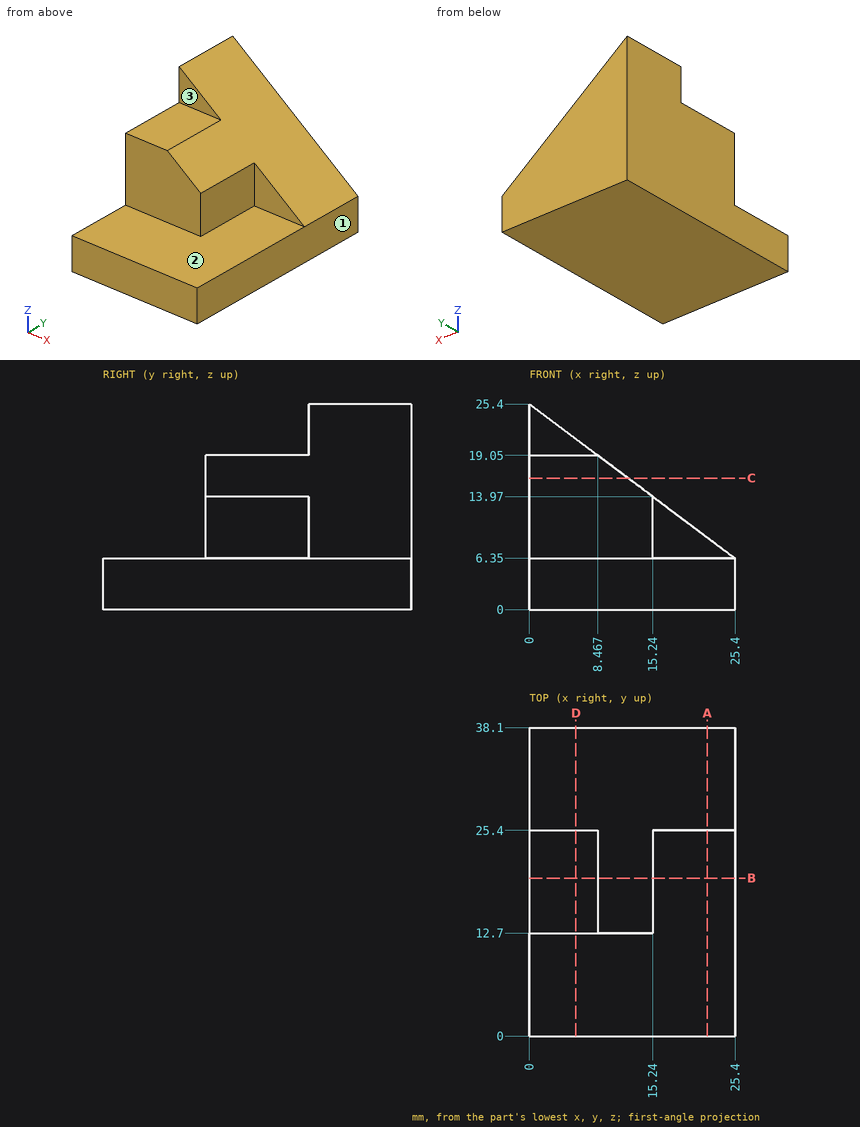
Could you check a few things on this drawing? It's one solid part, dimensions in mm from its lowest x, y, z. A direction names the side the tool comes from. Coordinates: 2 decimals unless noted, no trailing zeros. Loops run counter-clockwise (first coordinate to the right, second up) from the corner with the lowest first, then second, coordinate; pieces in that order, holes last. Notation, with made-up numbers: (89, 76.5) - (110, 76.5) arc R6 ccw to (110, 82.5) - close; hole circle Ø3 at (20, 43). An arc over 180 degrees is marked (long way). Return JSON: item names as keys, results as strings. Group by question number.
Item 1: If we section it at D-D on x = 5.75: Write out the boundary of the cut face in (y, z).
Item 2: Will these pins go through, and if not, where does the flat tip stop? P1, Ø7, axis at x = 4.5, z = 21.5, coming from the -Y side; P2, Ø3, axis at x = 13, y = 10, coming from the +Z side; P3, Ø7, axis at x = 5, y = 19.5, coming from the +Z side.
Item 3: If we section it at C-C on z = 16.25: Write out the boundary of the cut face in (x, y), and give its area (3 significant figures).
Item 4: I need wall thicknesses on line 1 (Y direction, x = 2.5, z = 8.5); line 2 (Z direction, x = 5.25, y = 7); line 3 (Z direction, x = 7.75, y = 16.5). Which ranges of each line are inside material? Lowest first, please. Write a range as from..to.
Item 5: On a 3-axis mill with a long thin cutter (end or side, diameter ignored), from which of +Z, -Z, +X, -X, +Y, -Y can I reach the whole of each face in a straight line? I mean the marked faces 1, 2 and 3. Say none if no direction works.
Item 6: If we section it at A-A on x = 22: Write out the boundary of the cut face in (y, z).
Item 7: If we section it at B-B on y = 19.5: Write out the boundary of the cut face in (x, z), and give its area (3 significant figures).
Calculated:
{
 "1": {"outline": "(0, 0) - (38.1, 0) - (38.1, 21.09) - (25.4, 21.09) - (25.4, 19.05) - (12.7, 19.05) - (12.7, 6.35) - (0, 6.35) - close"},
 "2": {"P1": "stops at y = 12.7", "P2": "stops at z = 6.35", "P3": "stops at z = 19.05"},
 "3": {"outline": "(0, 12.7) - (12.2, 12.7) - (12.2, 38.1) - (0, 38.1) - close", "area": "310 mm^2"},
 "4": {"line 1": "y = 12.7..38.1", "line 2": "z = 0..6.35", "line 3": "z = 0..19.05"},
 "5": {"face 1": "+Z, -Z, +X, +Y, -Y", "face 2": "+Z, +X, -Y", "face 3": "+Z, +X, -X, -Y"},
 "6": {"outline": "(0, 0) - (38.1, 0) - (38.1, 8.9) - (25.4, 8.9) - (25.4, 6.35) - (0, 6.35) - close"},
 "7": {"outline": "(0, 0) - (25.4, 0) - (25.4, 6.35) - (15.24, 6.35) - (15.24, 13.97) - (8.47, 19.05) - (0, 19.05) - close", "area": "338 mm^2"}
}
